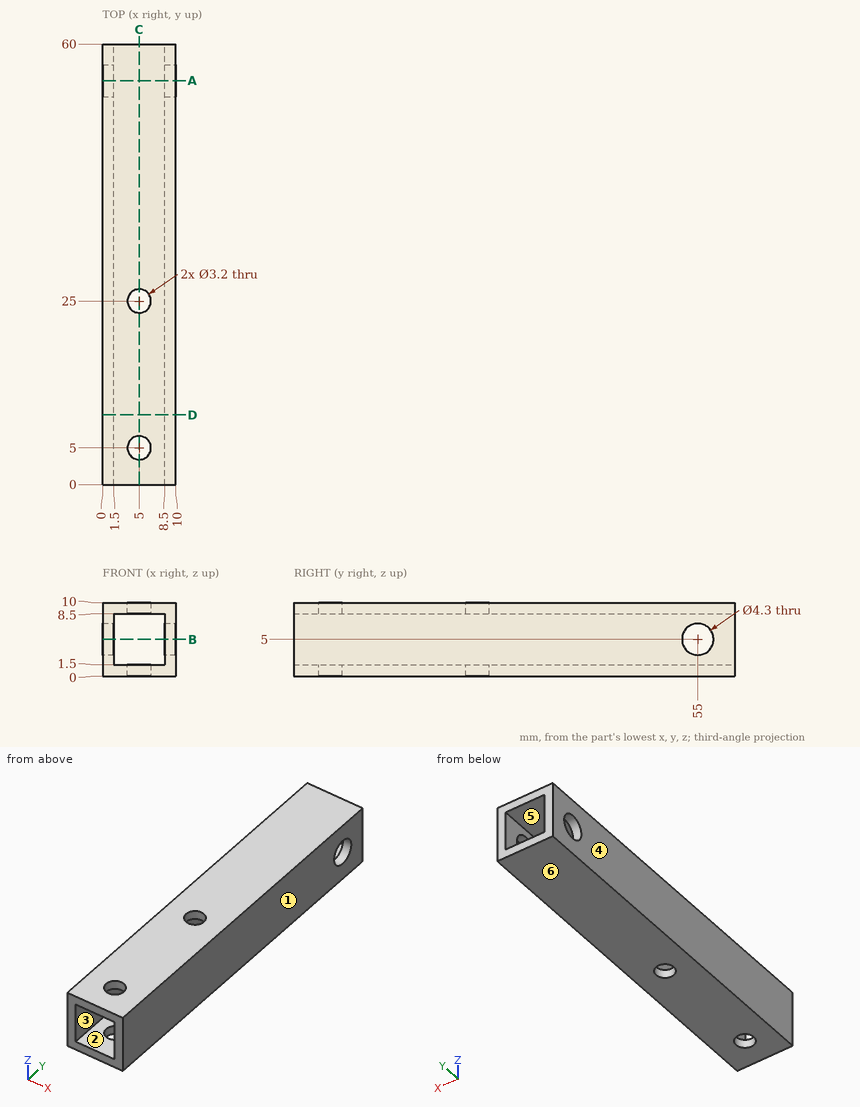
Input: dimensioned drawing with shaded views. Units: mm. Origin: part minimum x, y, z. A direction names the side the tool comes from. Coordinates: 2 decimals unless noted, no trailing zeros. Loops run counter-clockwise (first coordinate to the right, second up) from the corner with the lowest first, then second, coordinate; pieces in that order, holes last. Notation, with made-up numbers: M -17,65.5 L -10,65.5 A12 ccw -10,81.5 Z; hole C 83,-27 d11. An arc over 180 degrees is marked long. Use a Markdown table: item, result. Add a question column.
1) Section B-B, the plane z = 5. Return the cut outline in (x, y), plus the area to 3 significant figures.
2) Section A-A, the plane y = 55. Return the cut outline in (x, z), plus the area to 3 significant figures.
3) Section C-C, the plane x = 5. Return the cut outline in (y, z).
4) Set-up query: the marked faces 1 and 2. Return all of +Z, -Z, +X, -X, +Y, -Y with unobstructed straight access to the full face (end or side cutting, diameter ignored); none if empty.
5) Line query: L1, parallel to Y at x = 5, z = 0.75; L2, parallel to Z at x = 8, y = 11. Output: solid intervals per line, ascending. Write a range as from..to.
6) Section D-D, the plane y = 9.5. Return the cut outline in (x, z), plus the area to 3 significant figures.
7) Draft query along X for the marked faces 3, 4, 5 and 6. Return one class per face: +X half, -X half, draft (parallel to the pull), parting line (faces both ways), or undercut.
Answer below:
| question | item | result |
|---|---|---|
| 1 | outline | M 0,0 L 1.5,0 L 1.5,52.85 L 0,52.85 Z; M 0,57.15 L 1.5,57.15 L 1.5,60 L 0,60 Z; M 8.5,0 L 10,0 L 10,52.85 L 8.5,52.85 Z; M 8.5,57.15 L 10,57.15 L 10,60 L 8.5,60 Z |
| 1 | area | 167 mm2 |
| 2 | outline | M 0,0 L 10,0 L 10,2.85 L 8.5,2.85 L 8.5,1.5 L 1.5,1.5 L 1.5,2.85 L 0,2.85 Z; M 0,7.15 L 1.5,7.15 L 1.5,8.5 L 8.5,8.5 L 8.5,7.15 L 10,7.15 L 10,10 L 0,10 Z |
| 2 | area | 38.1 mm2 |
| 3 | outline | M 0,0 L 3.4,0 L 3.4,1.5 L 0,1.5 Z; M 0,8.5 L 3.4,8.5 L 3.4,10 L 0,10 Z; M 6.6,0 L 23.4,0 L 23.4,1.5 L 6.6,1.5 Z; M 6.6,8.5 L 23.4,8.5 L 23.4,10 L 6.6,10 Z; M 26.6,0 L 60,0 L 60,1.5 L 26.6,1.5 Z; M 26.6,8.5 L 60,8.5 L 60,10 L 26.6,10 Z |
| 4 | face 1 | +Z, -Z, +X, +Y, -Y |
| 4 | face 2 | +Y, -Y |
| 5 | L1 | 0..3.4, 6.6..23.4, 26.6..60 |
| 5 | L2 | 0..1.5, 8.5..10 |
| 6 | outline | M 0,0 L 10,0 L 10,10 L 0,10 Z; hole M 1.5,1.5 L 8.5,1.5 L 8.5,8.5 L 1.5,8.5 Z |
| 6 | area | 51.0 mm2 |
| 7 | face 3 | undercut |
| 7 | face 4 | -X half |
| 7 | face 5 | undercut |
| 7 | face 6 | draft |
